from build123d import *

# Parameters (mm, degrees)
BOSS_EXTRUDE1_DEPTH     = 53.5
BOSS_EXTRUDE2_START     = 32.75
BOSS_EXTRUDE2_DEPTH     = 10
BOSS_EXTRUDE3_DEPTH     = 2
FILLET1_R               = 10.75
FILLET2_R               = 14
FILLET3_R               = 1
CUT_EXTRUDE4_DEPTH      = 79.076260797
CUT_EXTRUDE5_DEPTH      = 61.840180017
CUT_EXTRUDE5_DEPTH_BACK = 61.840180017


# Some blends are built 0.0001 mm under size
with BuildPart() as part:
    # Sketch2 → Boss-Extrude1 (new body)
    with BuildSketch(Plane(origin=(0, 0, 0), x_dir=(1, 0, 0), z_dir=(0, 1, 0))):
        with BuildLine():
            Line((0, -12.75), (23.2, -12.75))
            ThreePointArc((23.2, -12.75), (35.95, 0), (23.2, 12.75))
            Line((23.2, 12.75), (0, 12.75))
            ThreePointArc((0, 12.75), (-12.75, 0), (0, -12.75))
        make_face()
        with BuildLine():
            ThreePointArc((23.2, -10.75), (33.95, 0), (23.2, 10.75))
            Line((23.2, 10.75), (0, 10.75))
            ThreePointArc((0, 10.75), (-10.75, 0), (0, -10.75))
            Line((0, -10.75), (23.2, -10.75))
        make_face(mode=Mode.SUBTRACT)
    extrude(amount=BOSS_EXTRUDE1_DEPTH)

    # Sketch2<3> → Boss-Extrude2 (add)
    with BuildSketch(Plane(origin=(0, 0, 0), x_dir=(1, 0, 0), z_dir=(0, 1, 0)).offset(BOSS_EXTRUDE2_START)):
        with BuildLine():
            Line((0, -10.75), (23.2, -10.75))
            ThreePointArc((23.2, -10.75), (33.95, 0), (23.2, 10.75))
            Line((23.2, 10.75), (0, 10.75))
            ThreePointArc((0, 10.75), (-10.75, 0), (0, -10.75))
        make_face()
    extrude(amount=BOSS_EXTRUDE2_DEPTH)

    # Sketch2<4> → Boss-Extrude3 (add)
    with BuildSketch(Plane(origin=(0, 0, 0), x_dir=(1, 0, 0), z_dir=(0, 1, 0))):
        with BuildLine():
            Line((0, 22.75), (23.2, 22.75))
            ThreePointArc((23.2, 22.75), (45.95, 0), (23.2, -22.75))
            Line((23.2, -22.75), (0, -22.75))
            ThreePointArc((0, -22.75), (-22.75, 0), (0, 22.75))
        make_face()
        with BuildLine():
            ThreePointArc((23.2, -12.75), (35.95, 0), (23.2, 12.75))
            Line((23.2, 12.75), (0, 12.75))
            ThreePointArc((0, 12.75), (-12.75, 0), (0, -12.75))
            Line((0, -12.75), (23.2, -12.75))
        make_face(mode=Mode.SUBTRACT)
    extrude(amount=BOSS_EXTRUDE3_DEPTH)

    # Fillet1
    fillet1_edges = [part.edges().sort_by_distance(p)[0] for p in [
        (11.6, 42.75, -10.75),
        (33.95, 42.75, 0),
        (11.6, 42.75, 10.75),
        (-10.75, 42.75, 0),
    ]]
    fillet(fillet1_edges, radius=FILLET1_R - 0.0001)  # a hair under: the kernel refuses the full size

    # Fillet2
    # the kernel refuses this fillet: 14 mm, written as the material it adds along each edge
    with BuildSketch(Plane(origin=(23.2, 2, 0), x_dir=(0, 0, 1), z_dir=(-1, 0, 0))) as fillet2_piece_1:
        with BuildLine():
            CenterArc((26.75, 13.416407865), FILLET2_R, 180, 73.398450401)
            Line((22.75, 0), (22.67, -0.268328157))
            ThreePointArc((22.67, -0.268328157), (17.75, -0.28), (12.75, -0.28))
            Line((12.75, -0.28), (12.47, 0))
            Line((12.47, 0), (12.47, 13.416407865))
            Line((12.47, 13.416407865), (12.75, 13.416407865))
        make_face()
    revolve(axis=Axis((23.2, 2, 0), (0, 1, 0)), revolution_arc=180)
    with BuildSketch(Plane(origin=(0, 2, 12.75), x_dir=(0, 1, 0), z_dir=(1, 0, 0)), Plane(origin=(23.2, 2, -12.75), x_dir=(0, 1, 0), z_dir=(-1, 0, 0))) as fillet2_piece_2:
        with BuildLine():
            CenterArc((13.416407865, 14), FILLET2_R, 196.601549599, 73.398450401)
            Line((0, 10), (-0.268328157, 9.92))
            ThreePointArc((-0.268328157, 9.92), (-0.28, 5), (-0.28, 0))
            Line((-0.28, 0), (0, -0.28))
            Line((0, -0.28), (13.416407865, -0.28))
            Line((13.416407865, -0.28), (13.416407865, 0))
        make_face()
    extrude(amount=23.2)
    with BuildSketch(Plane(origin=(0, 2, 0), x_dir=(0, 0, -1), z_dir=(1, 0, 0))) as fillet2_piece_3:
        with BuildLine():
            CenterArc((26.75, 13.416407865), FILLET2_R, 180, 73.398450401)
            Line((22.75, 0), (22.67, -0.268328157))
            ThreePointArc((22.67, -0.268328157), (17.75, -0.28), (12.75, -0.28))
            Line((12.75, -0.28), (12.47, 0))
            Line((12.47, 0), (12.47, 13.416407865))
            Line((12.47, 13.416407865), (12.75, 13.416407865))
        make_face()
    revolve(axis=Axis((0, 2, 0), (0, 1, 0)), revolution_arc=180)

    # Fillet3
    # the kernel refuses this fillet: 1 mm, written as the material it takes off along each edge
    with BuildSketch(Plane(origin=(0, 53.5, 10.75), x_dir=(0, 0, 1), z_dir=(1, 0, 0)), Plane(origin=(23.2, 53.5, -10.75), x_dir=(0, 0, -1), z_dir=(-1, 0, 0))) as fillet3_piece_1:
        with BuildLine():
            CenterArc((0.957377651, 1), FILLET3_R, 184.881694581, 85.118305419)
            Line((-0.038994884, 0.914901403), (-0.138632138, 0.906391544))
            ThreePointArc((-0.138632138, 0.906391544), (-0.1, 0.0001), (-0.1, 0))
            Line((-0.1, 0), (0, -0.1))
            Line((0, -0.1), (0.957377651, -0.1))
            Line((0.957377651, -0.1), (0.957377651, 0))
        make_face()
    extrude(amount=23.2, mode=Mode.SUBTRACT)
    with BuildSketch(Plane(origin=(0, 53.5, 0), x_dir=(0, 0, -1), z_dir=(1, 0, 0))) as fillet3_piece_2:
        with BuildLine():
            CenterArc((11.707377651, -1), FILLET3_R, 90, 85.118305419)
            Line((10.711005116, -0.914901403), (10.611367862, -0.906391544))
            ThreePointArc((10.611367862, -0.906391544), (10.65, -0.0001), (10.65, 0))
            Line((10.65, 0), (10.75, 0.1))
            Line((10.75, 0.1), (11.707377651, 0.1))
            Line((11.707377651, 0.1), (11.707377651, 0))
        make_face()
    revolve(axis=Axis((0, 53.5, 0), (0, 1, 0)), revolution_arc=180, mode=Mode.SUBTRACT)
    with BuildSketch(Plane(origin=(0, 53.5, 12.75), x_dir=(0, -1, 0), z_dir=(1, 0, 0))) as fillet3_piece_3:
        with BuildLine():
            CenterArc((FILLET3_R, FILLET3_R), FILLET3_R, 180, 90)
            Line((0, FILLET3_R), (0, 0))
            Line((0, 0), (FILLET3_R, 0))
        make_face()
    extrude(amount=23.2, mode=Mode.SUBTRACT)
    with BuildSketch(Plane(origin=(23.2, 53.5, 0), x_dir=(0, 0, 1), z_dir=(-1, 0, 0))) as fillet3_piece_4:
        with BuildLine():
            CenterArc((12.75 - FILLET3_R, -FILLET3_R), FILLET3_R, 0, 90)
            Line((12.75, -FILLET3_R), (12.75, 0))
            Line((12.75, 0), (12.75 - FILLET3_R, 0))
        make_face()
    revolve(axis=Axis((23.2, 53.5, 0), (0, 1, 0)), revolution_arc=180, mode=Mode.SUBTRACT)
    with BuildSketch(Plane(origin=(23.2, 53.5, -12.75), x_dir=(0, 0, 1), z_dir=(-1, 0, 0))) as fillet3_piece_5:
        with BuildLine():
            CenterArc((FILLET3_R, -FILLET3_R), FILLET3_R, 90, 90)
            Line((0, -FILLET3_R), (0, 0))
            Line((0, 0), (FILLET3_R, 0))
        make_face()
    extrude(amount=23.2, mode=Mode.SUBTRACT)
    with BuildSketch(Plane(origin=(0, 53.5, 0), x_dir=(0, 0, -1), z_dir=(1, 0, 0))) as fillet3_piece_6:
        with BuildLine():
            CenterArc((12.75 - FILLET3_R, -FILLET3_R), FILLET3_R, 0, 90)
            Line((12.75 - FILLET3_R, 0), (12.75, 0))
            Line((12.75, 0), (12.75, -FILLET3_R))
        make_face()
    revolve(axis=Axis((0, 53.5, 0), (0, 1, 0)), revolution_arc=180, mode=Mode.SUBTRACT)
    with BuildSketch(Plane(origin=(0, 2, -22.75), x_dir=(0, 0.30962089103713925, 0.9508600863604318), z_dir=(1, 0, 0)), Plane(origin=(23.2, 2, 22.75), x_dir=(0, 0.30962089103713925, -0.9508600863604318), z_dir=(-1, 0, 0))) as fillet3_piece_7:
        with BuildLine():
            CenterArc((0.726159611, 0.99968645), FILLET3_R, 198.036385117, 70.528779366)
            Line((-0.224700475, 0.690065559), (0, 0))
            ThreePointArc((0, 0), (0.350559812, 0.004389695), (0.701119624, 0))
        make_face()
    extrude(amount=23.2, mode=Mode.SUBTRACT)
    with BuildSketch(Plane(origin=(0, 2, 0), x_dir=(0, 0, 1), z_dir=(1, 0, 0))) as fillet3_piece_8:
        with BuildLine():
            CenterArc((21.75, 0.725727759), FILLET3_R, 289.471220634, 70.528779366)
            Line((22.75, 0.725727759), (22.75, 0))
            ThreePointArc((22.75, 0), (22.415307525, -0.104366656), (22.083333333, -0.217081283))
        make_face()
    revolve(axis=Axis((0, 2, 0), (0, -1, 0)), revolution_arc=180, mode=Mode.SUBTRACT)
    with BuildSketch(Plane(origin=(23.2, 2, 0), x_dir=(0, 0, -1), z_dir=(-1, 0, 0))) as fillet3_piece_9:
        with BuildLine():
            CenterArc((21.75, 0.725727759), FILLET3_R, 289.471220634, 70.528779366)
            Line((22.75, 0.725727759), (22.75, 0))
            ThreePointArc((22.75, 0), (22.415307525, -0.104366656), (22.083333333, -0.217081283))
        make_face()
    revolve(axis=Axis((23.2, 2, 0), (0, -1, 0)), revolution_arc=180, mode=Mode.SUBTRACT)
    with BuildSketch(Plane(origin=(23.2, 53.5, 0), x_dir=(0, 0, 1), z_dir=(-1, 0, 0))) as fillet3_piece_10:
        with BuildLine():
            CenterArc((11.707377651, -1), FILLET3_R, 90, 85.118305419)
            Line((10.711005116, -0.914901403), (10.611367862, -0.906391544))
            ThreePointArc((10.611367862, -0.906391544), (10.65, -0.0001), (10.65, 0))
            Line((10.65, 0), (10.75, 0.1))
            Line((10.75, 0.1), (11.707377651, 0.1))
            Line((11.707377651, 0.1), (11.707377651, 0))
        make_face()
    revolve(axis=Axis((23.2, 53.5, 0), (0, 1, 0)), revolution_arc=180, mode=Mode.SUBTRACT)

    # Sketch4 → Cut-Extrude4 (cut, through all)
    with BuildSketch(Plane.XY.offset(-10.75)):
        with BuildLine():
            Line((13.6, 0), (9.6, 0))
            Line((9.6, 0), (9.6, 1.331324862))
            ThreePointArc((9.6, 1.331324862), (11.6, 5.331324862), (13.6, 1.331324862))
            Line((13.6, 1.331324862), (13.6, 0))
        make_face()
    extrude(amount=-CUT_EXTRUDE4_DEPTH, mode=Mode.SUBTRACT)

    # Sketch3 → Cut-Extrude5 (cut, two sides: drawn at the far end of the back side and taken through both)
    with BuildSketch(Plane.XZ.offset(-32.75).offset(-CUT_EXTRUDE5_DEPTH_BACK)):
        with BuildLine():
            Line((9.2, 2.3), (14.2, 2.3))
            ThreePointArc((14.2, 2.3), (16.5, 0), (14.2, -2.3))
            Line((14.2, -2.3), (9.2, -2.3))
            ThreePointArc((9.2, -2.3), (6.9, 0), (9.2, 2.3))
        make_face()
    extrude(amount=CUT_EXTRUDE5_DEPTH + CUT_EXTRUDE5_DEPTH_BACK, mode=Mode.SUBTRACT)


solid = part.part
Verification items for the finished model (mm, model axes). A direction names the side the tool comes from. Coordinates: 2 decimals unless noted, no trailing zeros. Order: outer loops, then holes, each group sorted by start corner. A loop starts at its lowest first (then second) coordinate and runs counter-clockwise, first axis right, second up. Notation, with made-up numbers: M 66.5,29.5 L 125.5,29.5 A17 ccw 125.5,56.5 Z; hole C 62,5 d3. An arc over 180 degrees is marked long. One line per item, written item: value. Start each with the question number.
Item 1: Sectioned sample at C-C on y = 4.5. Record the cut outline in (x, z), then the cut area to 3 significant figures.
Item 2: Mould release check, pull along Z, two halves, no side actions. Record for faces 1 (the flat face through (12, 38, -2.3)), 2 (the cylindrical face through (11.438, 7.235, 15.389)), 3 (the cylindrical face through (11.52, 5.33, -15.33)): pulls with the +Z half, pulls with the -Z half, needs draft (parallel to the pull), parting line crosses it, or undercut.
Item 3: Sectioned sample at D-D on y = 40. Record the cut outline in (x, z), then the cut area to 3 significant figures.
Item 4: Sectioned sample at B-B on y = 23. Record the cut outline in (x, z).
Item 5: Sectioned sample at A-A on x = 11.6. Record the cut outline in (y, z), then the cut area to 3 significant figures.
Item 6: Access from +Z, -Z, +X, -X, +Y, -Y to the whole of each face (thin tool, end or side, straight path). Record for faces 4 (the flat face through (12, 16, -10.75)), 5 (the cylindrical face through (-12.747, 33.699, -0.28)), 6 (the cylindrical face through (6.9, 37.95, -0.05)).
Item 7: Depth check by flat-ended pin: P1, Ø1.5, axis at x = 0, y = 19.5, coming from the +Z side; P2, Ø7, axis at x = 16, y = 14, coming from the -Z side; P3, Ø5, axis at x = -3.5, z = 17.5, coming from the +Y side. Enter the tip coordinate at first touch or a pass-through.
Item 8: Thickness scan on probe 1 along Y at (x, z) = (37, 17); probe 2 along Z at (x, y) = (-5, 15); probe 3 along Z at (x, y) = (0, 49.5). Record the ranges inside material, lowest first.
Calculated:
1. outline: M 0,-17.98 L 9.74,-17.98 L 9.74,-10.75 L 0,-10.75 A10.75 cw 0,10.75 L 23.2,10.75 A10.75 cw 23.2,-10.75 L 13.46,-10.75 L 13.46,-17.98 L 23.2,-17.98 A17.98 ccw 23.2,17.98 L 0,17.98 A17.98 ccw Z
1. area: 962 mm^2
2. face 1: undercut
2. face 2: pulls with the +Z half
2. face 3: needs draft
3. outline: M 0,-12.75 L 23.2,-12.75 A12.75 ccw 23.2,12.75 L 0,12.75 A12.75 ccw Z; hole M 9.2,-2.3 L 14.2,-2.3 A2.3 ccw 14.2,2.3 L 9.2,2.3 A2.3 ccw Z
3. area: 1,060 mm^2
4. outline: M 0,-12.75 L 23.2,-12.75 A12.75 ccw 23.2,12.75 L 0,12.75 A12.75 ccw Z; hole M 0,-10.75 L 23.2,-10.75 A10.75 ccw 23.2,10.75 L 0,10.75 A10.75 ccw Z
5. outline: M 0,10.75 L 32.75,10.75 L 32.75,2.3 L 43,2.3 A10.75 cw 52.59,10.71 A1 ccw 53.5,11.71 L 53.5,11.75 A1 ccw 52.5,12.75 L 15.42,12.75 A14 cw 2.22,22.08 A1 ccw 1.27,22.75 L 0,22.75 Z; M 5.33,-17.04 A14 cw 15.42,-12.75 L 52.5,-12.75 A1 ccw 53.5,-11.75 L 53.5,-11.71 A1 ccw 52.59,-10.71 A10.75 cw 43,-2.3 L 32.75,-2.3 L 32.75,-10.75 L 5.33,-10.75 Z
5. area: 490 mm^2
6. face 4: -Y
6. face 5: -X, +Y
6. face 6: +Y, -Y
7. P1: z = 12.75
7. P2: z = -13.64
7. P3: y = 7.29
8. probe 1: 0 to 2.28
8. probe 2: -11.74 to -9.52, 9.52 to 11.74
8. probe 3: -12.75 to -9.98, 9.98 to 12.75
